from build123d import *

# Parameters (mm, degrees)
F0_R     = 12.5
F0_R_2   = 7.5
F1_DEPTH = 25


with BuildPart() as f1:
    # F0 (on Top) → F1 (new body)
    with BuildSketch(Plane.XY):
        Polygon((80, 114.432458), (-37.5, 114.432458), (-37.5, 56.732458), (0, 56.732458), (0, 39.232458), (-70, 39.232458), (-70, -73.267542), (-50, -73.267542), (-25, -73.267542), (0, -73.267542), (35.415397, -73.267542), (57.5, -20.567542), (57.5, 41.932458), (80, 41.932458), (80, 96.932458), align=None)
        with Locations((-47.084603, -58.267542)):
            Circle(F0_R, mode=Mode.SUBTRACT)
        with Locations((-22.084603, -33.267542)):
            Circle(F0_R, mode=Mode.SUBTRACT)
        with Locations((0, -8.267542)):
            Circle(F0_R, mode=Mode.SUBTRACT)
        with Locations((-22.5, 96.932458)):
            Circle(F0_R_2, mode=Mode.SUBTRACT)
        with Locations((2.5, 96.932458)):
            Circle(F0_R_2, mode=Mode.SUBTRACT)
        with Locations((22.5, 96.932458)):
            Circle(F0_R_2, mode=Mode.SUBTRACT)
        with Locations((42.5, 96.932458)):
            Circle(F0_R_2, mode=Mode.SUBTRACT)
        with Locations((62.5, 96.932458)):
            Circle(F0_R_2, mode=Mode.SUBTRACT)
        with Locations((0, -8.267542)):
            Circle(F0_R)
        with Locations((-22.084603, -33.267542)):
            Circle(F0_R)
    extrude(amount=F1_DEPTH)


solid = f1.part
Design review of the part built by this model. Coordinates are the model's own, in mm. A direction names the side the tool comes from. Coordinates: 2 decimals unless noted, no trailing zeros. Write each loop counter-clockwise with the first axis right and the second up, starting at its lowest first coordinate (ties: lowest second). Pieces come first, ordered by that corner, then holes. Notation, with made-up numbers: (-11.75, 45) - (29.25, 45) arc R24 cw to (29.25, 72) - close; hole circle Ø9 at (51.5, -26.75). An arc over 180 degrees is marked (long way). One line per item, written item: value.
1) To check wall thickness, follow probe 1 along X at (y, z) = (94, 5); probe 2 along X at (y, z) = (100.5, 1.5); probe 3 along Y at (x, z) = (23, 2). State the ranges of each line that lie inside material, in increasing order.
Answer sheet:
probe 1: x = -37.5 to -29.4, -15.6 to -4.4, 9.4 to 15.6, 29.4 to 35.6, 49.4 to 55.6, 69.4 to 80
probe 2: x = -37.5 to -29.1, -15.9 to -4.1, 9.1 to 15.9, 29.1 to 35.9, 49.1 to 55.9, 69.1 to 80
probe 3: y = -73.27 to 89.45, 104.42 to 114.43
2) Add section A-A (x = -22.5). State the section outline as (y, z) points, plus the area to 3 significant figures.
Answer sheet:
outline: (-73.27, 0) - (39.23, 0) - (39.23, 25) - (-73.27, 25) - close; (56.73, 0) - (89.43, 0) - (89.43, 25) - (56.73, 25) - close; (104.43, 0) - (114.43, 0) - (114.43, 25) - (104.43, 25) - close
area: 3,880 mm2
3) For faces 4 (the face through (-37.5, 86, 12)), 5 (the face through (-35, 39.232, 12)), 6 (the face through (4, 22, 0)), 7 (the face through (69, 41.932, 12)), list the 3-axis set-ups (+Z, -Z, +X, -X, +Y, -Y) from which the entire face can be reached by the end or side of a thin tool; tool diameter is ignored.
Answer sheet:
face 4: +Z, -Z, -X, +Y
face 5: +Z, -Z, -X
face 6: -Z, +X, -X, +Y, -Y
face 7: +Z, -Z, +X, -Y
4) Insertion check: pin 1 (13.5 mm diameter, centred on x = 22.5, y = 96.93, fed in from +Z); pin 2 (7.5 mm diameter, centred on y = 92, z = 18, fed in from -X); pin 3 (14 mm diameter, centred on y = 49, z = 13, fed in from -X); pin 4 (7.5 mm diameter, centred on y = 14.5, z = 18.5, fed in from +X). Each pin has a flat end and moves straight along its axis. Give the tip position at first contact, or say it passes through.
Answer sheet:
pin 1: passes through
pin 2: stops at x = -37.5
pin 3: stops at x = 0
pin 4: stops at x = 57.5
5) Add section D-D (y = 51). State the section outline as (x, z) points, plus the area to 3 significant figures.
Answer sheet:
outline: (0, 0) - (80, 0) - (80, 25) - (0, 25) - close
area: 2,000 mm2
6) Add section B-B (x = 2.5). State the section outline as (y, z) points.
Answer sheet:
outline: (-73.27, 0) - (89.43, 0) - (89.43, 25) - (-73.27, 25) - close; (104.43, 0) - (114.43, 0) - (114.43, 25) - (104.43, 25) - close
7) Add section C-C (z = 23). State the section outline as (x, y) points.
Answer sheet:
outline: (-70, -73.27) - (35.42, -73.27) - (57.5, -20.57) - (57.5, 41.93) - (80, 41.93) - (80, 114.43) - (-37.5, 114.43) - (-37.5, 56.73) - (0, 56.73) - (0, 39.23) - (-70, 39.23) - close; hole circle Ø25 at (-47.08, -58.27); hole circle Ø15 at (-22.5, 96.93); hole circle Ø15 at (2.5, 96.93); hole circle Ø15 at (22.5, 96.93); hole circle Ø15 at (42.5, 96.93); hole circle Ø15 at (62.5, 96.93)
8) Mouldability with a two-part tool opening along Y and no side actions: class faces 1 (the face through (46, 90.3, 12.3)), 2 (the face through (-18, -73.268, 12)), 3 (the face through (57.5, 10, 12)) as +Y half, -Y half, draft (parallel to the pull), parting line (faces both ways), or undercut.
Answer sheet:
face 1: undercut
face 2: -Y half
face 3: draft
